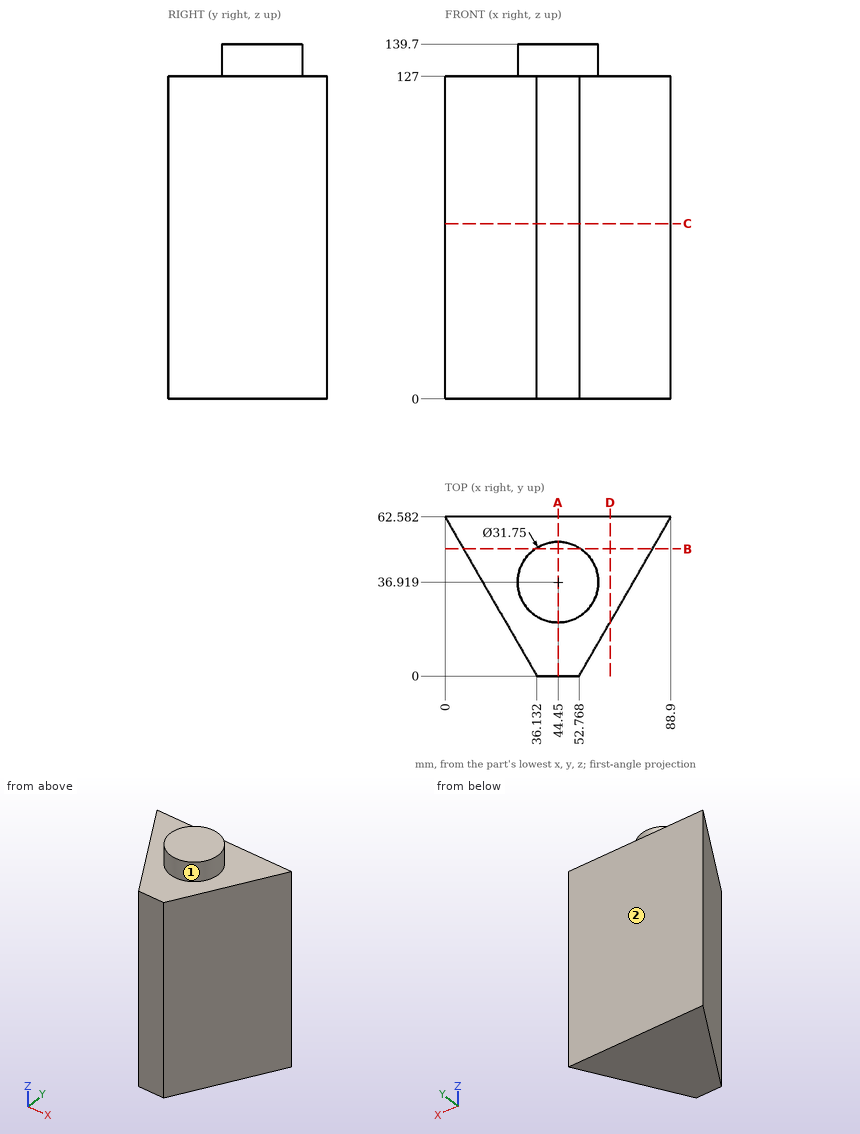
Here's the drawing with two shaded views (mm, measured from the low corner). I have some questions. A direction names the side the tool comes from. Round coordinates to 2 decimals unless told otherwise and drop trailing zeros. Loops run counter-clockwise (first coordinate to the right, second up) from the corner with the lowest first, then second, coordinate; pieces in that order, holes last. Notation, with made-up numbers: M -18,53 L 11,53 A28 ccw 11,72 Z; hole C 67.5,52 d2. An arc over 180 degrees is marked long. Answer as a JSON object with one key per item and string values. Group by question number.
Q1. Please list where these lines run through material, in increasing order: L1, parallel to Z at x = 58.5, y = 55.5; L2, parallel to X at y = 40.5, z = 88; L3, parallel to X at y = 60.5, z = 60.
Q2. Imagine slicing it at D-D, the plane x = 65. Please give me the cut outline in (y, z).
Q3. Imagine slicing it at C-C, the plane z = 69. Please give me the cut outline in (x, y).
Q4. Imagine slicing it at B-B, the plane y = 50. Please give me the cut outline in (x, z).
Q5. On a 3-axis mill with a long thin cutter (end or side, diameter ignored), from which of +Z, -Z, +X, -X, +Y, -Y can I reach the whole of each face in a straight line? I mean the marked faces 1 and 2. Say none if no direction works.
Q6. Will these pins go through, and if not, where does the flat tip stop? pin 1 (1.5 mm diameter, centred on y = 10.5, z = 99.5, fed in from -X); pin 2 (12 mm diameter, centred on x = 14.5, y = 47.5, fed in from -Z); pin 3 (1.5 mm diameter, centred on y = 48.5, z = 14.5, fed in from +X); pin 4 (1 mm diameter, centred on x = 14, y = 47, fed in from +Z).
Q7. Imagine slicing it at A-A, the plane x = 44.45. Please give me the cut outline in (y, z), then the cut area to 3 significant figures.
Findings:
{
 "1": {"L1": "z = 0 to 127", "L2": "x = 12.75 to 76.15", "L3": "x = 1.2 to 87.7"},
 "2": {"outline": "M 21.19,0 L 62.58,0 L 62.58,127 L 21.19,127 Z"},
 "3": {"outline": "M 0,62.58 L 36.13,0 L 52.77,0 L 88.9,62.58 Z"},
 "4": {"outline": "M 7.26,0 L 81.64,0 L 81.64,127 L 53.44,127 L 53.44,139.7 L 35.46,139.7 L 35.46,127 L 7.26,127 Z"},
 "5": {"face 1": "+Z", "face 2": "+Z, -Z, +X, -X, +Y"},
 "6": {"pin 1": "stops at x = 29.64", "pin 2": "stops at z = 0", "pin 3": "stops at x = 81.2", "pin 4": "stops at z = 127"},
 "7": {"outline": "M 0,0 L 62.58,0 L 62.58,127 L 52.79,127 L 52.79,139.7 L 21.04,139.7 L 21.04,127 L 0,127 Z", "area": "8,350 mm2"}
}
